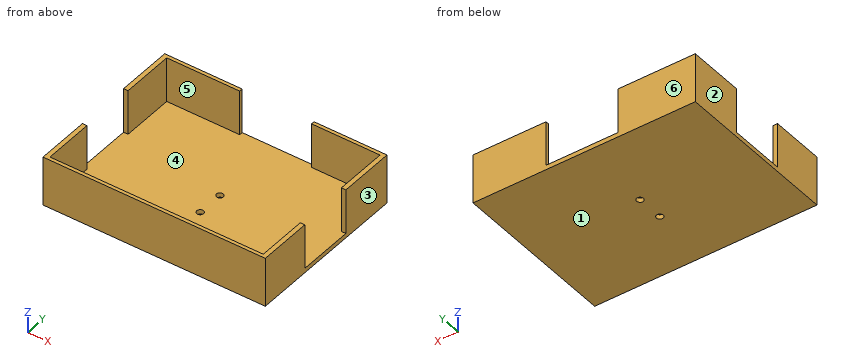
Autodesk Fusion 360 part; units mm, degrees
sketch "Szkic1" plane through (0, 0, 0) normal (0, 0, 1) x (1, 0, 0)
  line L0 (0, 0) -> (99, 0)
  line L1 (99, 0) -> (99, 74)
  line L2 (99, 74) -> (0, 74)
  line L3 (0, 74) -> (0, 0)
  line L4 (0, 74) -> (2, 74)
  line L5 (2, 74) -> (2, 0)
  line L6 (0, 74) -> (0, 72.5)
  line L7 (0, 72.5) -> (99, 72.5)
  line L8 (0, 0) -> (0, 1.5)
  line L9 (0, 1.5) -> (99, 1.5)
  line L10 (99, 0) -> (97, 0)
  line L11 (97, 0) -> (97, 74)
  line L12 (0, 74) -> (34.5, 74)
  line L13 (34.5, 74) -> (34.5, 72.5)
  line L14 (66.5, 74) -> (66.5, 72.5)
  line L15 (0, 74) -> (0, 49)
  line L16 (0, 49) -> (2, 49)
  line L17 (0, 49) -> (0, 24)
  line L18 (0, 24) -> (2, 24)
  line L19 (99, 74) -> (99, 49)
  line L20 (99, 49) -> (97, 49)
  line L21 (99, 49) -> (99, 24)
  line L22 (99, 24) -> (97, 24)
  line L23 (49.5, 0) -> (49.5, 28) construction
  line L24 (49.5, 28) -> (49.5, 40) construction
  circle A0 centre (49.5, 40) radius 1.5
  circle A1 centre (49.5, 28) radius 1.5
  point P0 (49.5, 0)
  dimension "d1" = 99
  dimension "d2" = 74
  dimension "d3" = 2
  dimension "d5" = 2
  dimension "d6" = 34.5
  dimension "d7" = 32
  dimension "d8" = 25
  dimension "d9" = 25
  dimension "d10" = 25
  dimension "d11" = 25
  dimension "d18" = 3
  dimension "d19" = 3
  dimension "d22" = 28
  dimension "d23" = 12
  dimension "d26" = 1.5
  dimension "d27" = 1.5
extrude "Wyciągnięcie proste1" add sketch "Szkic1" along normal blind 22 contours L0 L3 L5 L8 L9 | L0 L5 L9 L11 | L3 L5 L9 L18 | L0 L1 L9 L10 L11 | L1 L9 L11 L22 | L3 L5 L7 L15 L16 | L2 L3 L4 L5 L6 L7 L12 L15 | L1 L7 L11 L19 L20 | L2 L5 L7 L12 L13 | L1 L2 L7 L11 L19 | L2 L7 L11 L14 makes body 1 at (33, 0, 7.3333) makes body 2 at (88.1667, 74, 14.6667) makes body 3 at (23, 74, 7.3333)
extrude "Wyciągnięcie proste2" add sketch "Szkic1" along normal blind 1 separate body contours L5 L7 L9 L11 | L3 L5 L16 L17 L18 | L1 L11 L20 L21 L22 | L2 L7 L13 L14 | A0 | A1 makes body 4
combine "Kombinacja1" operation add target body 4 tool bodies 3 1 2
extrude "Wyciągnięcie proste3" cut sketch "Szkic1" along normal blind 6 contours A0 | A1 bodies 4
extrude "Wyciągnięcie proste4" add 1 faces at (49.4799, 9.8337, 1) along direction (0, 0, 1) blind 1 on bodies 4 bodies 4
Here's how the part is built. I have some questions about the finished solid (model axes, mm). Face numbers are marked on the shaded views. A direction names the side the tool comes from. Coordinates: 2 decimals unless noted, no trailing zeros. Order: outer loops, then holes, each group sorted by start corner. A loop starts at its lowest first (then second) coordinate and runs counter-clockwise, first axis right, second up.
Item 1: If we section it at D-D, the plane y = 15: List the corners of the cut face in (x, z) for me, then the cut area to 3 significant figures.
Response values:
outline: (0, 0) - (99, 0) - (99, 22) - (97, 22) - (97, 2) - (2, 2) - (2, 22) - (0, 22) - close
area: 278 mm2
Item 2: If we section it at A-A, the plane y = 40: List the corners of the cut face in (x, z) for me.
Response values:
outline: (0, 0) - (48, 0) - (48, 2) - (0, 2) - close; (51, 0) - (99, 0) - (99, 2) - (51, 2) - close
Item 3: Thinking about a two-plate mould opening in X: for the marked faces 1, 2, 3 and 4, which applies, pulls with the +X half, pulls with the -X half, needs draft (parallel to the pull), parting line crosses it, or undercut?
Response values:
face 1: needs draft
face 2: pulls with the -X half
face 3: pulls with the +X half
face 4: undercut
Item 4: If we section it at B-B, the plane z = 8.25: List the corners of the cut face in (x, y) for me, then the cut area to 3 significant figures.
Response values:
outline: (0, 0) - (99, 0) - (99, 24) - (97, 24) - (97, 1.5) - (2, 1.5) - (2, 24) - (0, 24) - close; (0, 49) - (2, 49) - (2, 72.5) - (34.5, 72.5) - (34.5, 74) - (0, 74) - close; (66.5, 72.5) - (97, 72.5) - (97, 49) - (99, 49) - (99, 74) - (66.5, 74) - close
area: 433 mm2
Item 5: I'm going to push a flat-ended pin straight in: pin 1 Ø22 at (x, y) = (32, 50) entering from +Z. Where does the tip first touch, or does it pass through?
Response values:
pin 1: stops at z = 2
Item 6: If we section it at C-C, the plane x = 49.5: List the corners of the cut face in (y, z) for me, then the cut area to 3 significant figures.
Response values:
outline: (0, 0) - (26.5, 0) - (26.5, 2) - (1.5, 2) - (1.5, 22) - (0, 22) - close; (29.5, 0) - (38.5, 0) - (38.5, 2) - (29.5, 2) - close; (41.5, 0) - (74, 0) - (74, 2) - (41.5, 2) - close
area: 166 mm2
Item 7: I need wall thicknesses on probe 1 along Y at (x, z) = (49.5, 1.2); probe 2 along X at (y, z) = (15, 11.5); probe 3 along X at (y, z) = (40, 0.4). Which ranges of each line are inside material? Lowest first, please.
Response values:
probe 1: y = 0 to 26.5, 29.5 to 38.5, 41.5 to 74
probe 2: x = 0 to 2, 97 to 99
probe 3: x = 0 to 48, 51 to 99
Item 8: Which directions (+Z, -Z, +X, -X, +Y, -Y) give clear straight access to the entire face, cutting with the end or side of a thin tool? Please do the marked faces 5 and 6.
Response values:
face 5: +Z
face 6: +Z, -Z, +X, -X, +Y
